Can you work these out from the model? Positions are in its coordinate system, mm. Round coordinates to 2 decimals unless told otherwise and drop trailing zeros. Loops run counter-clockwise (first coordinate to the right, second up) from the corner with the lowest first, then second, coordinate; pieces in that order, holes last. Notation, with made-up numbers: (28.25, 74) -> (35.25, 74) arc R21 ccw to (35.25, 113) -> close; hole circle Ø8 at (82.25, 84). An arc over 180 degrees is marked (long way). Use a Markdown table: item, result.
from build123d import *

# Parameters (mm, degrees)
SKETCH1_R           = 12.525
SKETCH1_R_2         = 1.55
SKETCH1_R_3         = 2.5
SKETCH1_R_4         = 2.25
SKETCH1_R_5         = 2
SKETCH1_W           = 8
SKETCH1_H           = 5
BOSS_EXTRUDE1_DEPTH = 1.5


with BuildPart() as part:
    # Sketch1 → Boss-Extrude1 (new body)
    with BuildSketch(Plane(origin=(0, 0, 0), x_dir=(1, 0, 0), z_dir=(0, 1, 0))):
        with BuildLine():
            Line((44.790320824, 89.722222222), (71.664513318, 35.555555556))
            ThreePointArc((71.664513318, 35.555555556), (0, -80), (-71.664513318, 35.555555556))
            Line((-71.664513318, 35.555555556), (-44.790320824, 89.722222222))
            ThreePointArc((-44.790320824, 89.722222222), (0, 117.5), (44.790320824, 89.722222222))
        make_face()
        Circle(SKETCH1_R, mode=Mode.SUBTRACT)
        with Locations((-17.5, -10.103629711)):
            Circle(SKETCH1_R_2, mode=Mode.SUBTRACT)
        with Locations((17.5, -10.103629711)):
            Circle(SKETCH1_R_2, mode=Mode.SUBTRACT)
        with Locations((0, 20.207259422)):
            Circle(SKETCH1_R_2, mode=Mode.SUBTRACT)
        with Locations((0, 67.5)):
            Circle(SKETCH1_R_3, mode=Mode.SUBTRACT)
        with Locations((40, 67.5)):
            Circle(SKETCH1_R_4, mode=Mode.SUBTRACT)
        with Locations((70, 0)):
            Circle(SKETCH1_R_4, mode=Mode.SUBTRACT)
        with Locations((56.631189606, -41.14496766)):
            Circle(SKETCH1_R_4, mode=Mode.SUBTRACT)
        with Locations((21.631189606, -66.573956141)):
            Circle(SKETCH1_R_4, mode=Mode.SUBTRACT)
        with Locations((-21.631189606, -66.573956141)):
            Circle(SKETCH1_R_4, mode=Mode.SUBTRACT)
        with Locations((-56.631189606, -41.14496766)):
            Circle(SKETCH1_R_4, mode=Mode.SUBTRACT)
        with Locations((-70, 0)):
            Circle(SKETCH1_R_4, mode=Mode.SUBTRACT)
        with Locations((28.284271247, 95.784271247)):
            Circle(SKETCH1_R_4, mode=Mode.SUBTRACT)
        with Locations((0, 107.5)):
            Circle(SKETCH1_R_4, mode=Mode.SUBTRACT)
        with Locations((-28.284271247, 95.784271247)):
            Circle(SKETCH1_R_4, mode=Mode.SUBTRACT)
        with Locations((-40, 67.5)):
            Circle(SKETCH1_R_4, mode=Mode.SUBTRACT)
        with Locations((-50.153461651, 44.654711284)):
            Circle(SKETCH1_R_4, mode=Mode.SUBTRACT)
        with Locations((-60.306923303, 21.809422569)):
            Circle(SKETCH1_R_4, mode=Mode.SUBTRACT)
        with Locations((50.153461651, 44.654711284)):
            Circle(SKETCH1_R_4, mode=Mode.SUBTRACT)
        with Locations((60.306923303, 21.809422569)):
            Circle(SKETCH1_R_4, mode=Mode.SUBTRACT)
        with Locations((17.859623375, -30.100396225)):
            Circle(SKETCH1_R_5, mode=Mode.SUBTRACT)
        with Locations((-23.249483938, 26.162215055)):
            Circle(SKETCH1_R_5, mode=Mode.SUBTRACT)
        with Locations((0, 47.5)):
            Rectangle(SKETCH1_W, SKETCH1_H, mode=Mode.SUBTRACT)
        with Locations((-1.994503305, -58.420364393)):
            Rectangle(SKETCH1_W, SKETCH1_H, mode=Mode.SUBTRACT)
        with Locations((-34.37581539, 50)):
            Rectangle(SKETCH1_W, SKETCH1_H, mode=Mode.SUBTRACT)
        with Locations((34.136464886, 49.290075758)):
            Rectangle(SKETCH1_W, SKETCH1_H, mode=Mode.SUBTRACT)
        with Locations((54.012994775, -0.420504721)):
            Rectangle(SKETCH1_W, SKETCH1_H, mode=Mode.SUBTRACT)
        with Locations((-56.673760324, -13.260168312)):
            Rectangle(SKETCH1_W, SKETCH1_H, mode=Mode.SUBTRACT)
        with Locations((-0.046638908, 98.711772009)):
            Rectangle(SKETCH1_W, SKETCH1_H, mode=Mode.SUBTRACT)
    extrude(amount=BOSS_EXTRUDE1_DEPTH)


solid = part.part
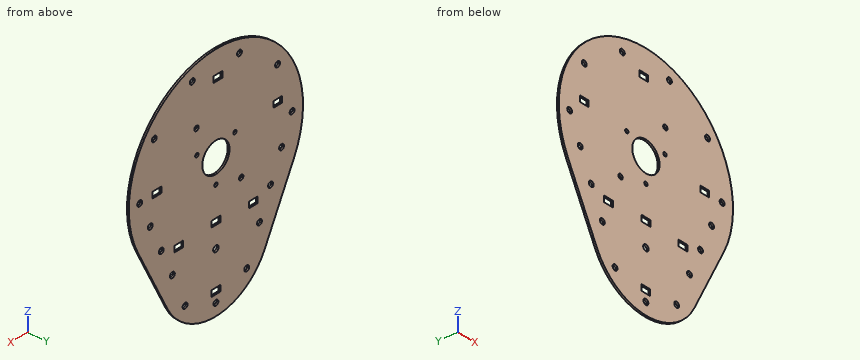
1. Will these pins go through, and if not, where does the flat tip stop? pin 1 Ø0.8 at (x, y) = (32.5, 0.5) entering from -Z; pin 2 Ø0.8 at (x, y) = (-32.5, 0.5) entering from +Z.
Answer sheet:
| item | result |
|---|---|
| pin 1 | stops at z = -105.84 |
| pin 2 | stops at z = 73.28 |
2. I want a section at A-A (z = -107.5). Please give me the cut outline in (x, y), plus the area to 4 significant figures.
Answer sheet:
| item | result |
|---|---|
| outline | (-30, 0) -> (-2.25, 0) -> (-2.25, 1.5) -> (-30, 1.5) -> close; (2.25, 0) -> (30, 0) -> (30, 1.5) -> (2.25, 1.5) -> close |
| area | 83.25 mm² |
3. I want a section at B-B (z = 0). Please give me the cut outline in (x, y) (3 decimals), plus the area to 3 significant figures.
Answer sheet:
| item | result |
|---|---|
| outline | (-80, 0) -> (-72.25, 0) -> (-72.25, 1.5) -> (-80, 1.5) -> close; (-67.75, 0) -> (-12.525, 0) -> (-12.525, 1.5) -> (-67.75, 1.5) -> close; (12.525, 0) -> (50.013, 0) -> (50.013, 1.5) -> (12.525, 1.5) -> close; (58.013, 0) -> (67.75, 0) -> (67.75, 1.5) -> (58.013, 1.5) -> close; (72.25, 0) -> (80, 0) -> (80, 1.5) -> (72.25, 1.5) -> close |
| area | 177 mm² |
4. I want a section at C-C (y = 0.6). State how many separate pieces and enclosed holes the cut face has, plus the area to 3 significant figures.
Answer sheet:
| item | result |
|---|---|
| separate pieces | 1 |
| enclosed holes | 29 |
| area | 22,600 mm² |
5. I need wall thicknesses on line 1 (X direction, y = 0.4, z = 0) (3 decimals); line 2 (X direction, y = 1, z = 67.5); line 3 (Z direction, x = -56, y = 0.7). Which ranges of each line are inside material? Lowest first, please.
Answer sheet:
| item | result |
|---|---|
| line 1 | x = -80 to -72.25, -67.75 to -12.525, 12.525 to 50.013, 58.013 to 67.75, 72.25 to 80 |
| line 2 | x = -42.94 to -23.68, -19.58 to 19.58, 23.68 to 42.94 |
| line 3 | z = -67.13 to 10.76, 15.76 to 38.99, 43.3 to 57.13 |
6. I want a section at D-D (z = -84). Please give me the cut outline in (x, y), plus the area to 3 significant figures.
Answer sheet:
| item | result |
|---|---|
| outline | (-47.63, 0) -> (47.63, 0) -> (47.63, 1.5) -> (-47.63, 1.5) -> close |
| area | 143 mm² |
